Autodesk Inventor part; units mm, degrees
ref_plane "YZ Plane" through (0, 0, 0) normal (1, 0, 0) x (0, 1, 0)
ref_plane "XZ Plane" through (0, 0, 0) normal (0, 1, 0) x (-1, 0, 0)
ref_plane "XY Plane" through (0, 0, 0) normal (0, 0, 1) x (1, 0, 0)
sketch "Szkic1" plane through (0, 0, 0) normal (0, 0, 1) x (1, 0, 0)
  line L0 (-106, 20) -> (0, 20)
  line L1 (-106, 20) -> (-106, -2)
  line L2 (-106, -2) -> (24.7184, -2)
  line L3 (24.7184, -2) -> (24.7184, 3)
  line L4 (24.7184, 3) -> (0, 20)
  circle A0 centre (8, 6.2) radius 2 construction
  circle A1 centre (8, 6.2) radius 2.25
  line L5 (-57.5, 18) -> (-45.5, 18)
  line L6 (-45.5, 18) -> (-45.5, 8)
  line L7 (-45.5, 8) -> (-57.5, 8)
  line L8 (-57.5, 8) -> (-57.5, 18)
  line L9 (-70, 12.4) -> (-70, 0) construction
  arc A2 (-86.6773, 8.9692) -> (-86.6773, 3.4308) centre (-92, 6.2) ccw construction
  arc A3 (-86, 3.7) -> (-86, 8.7) centre (-86, 6.2) ccw construction
  arc A4 (-86.2337, 3.7) -> (-86.6773, 3.4308) centre (-86.2337, 3.2) ccw construction
  line L10 (-86.2337, 3.7) -> (-86, 3.7) construction
  arc A5 (-86.6773, 8.9692) -> (-86.2337, 8.7) centre (-86.2337, 9.2) ccw construction
  line L11 (-86, 8.7) -> (-86.2337, 8.7) construction
  arc A6 (-86.375, 8.9243) -> (-86.375, 3.4757) centre (-92, 6.2) ccw
  arc A7 (-86.375, 3.4757) -> (-86.375, 8.9243) centre (-86, 6.2) ccw
  line L12 (-116, 20) -> (-106, 20)
  line L13 (-106, 20) -> (-106, -2)
  line L14 (-106, -2) -> (-116, -2)
  line L15 (-116, -2) -> (-116, 20)
  line L16 (-92, 6.2) -> (-92, -8.9) construction
  line L17 (-92, -8.9) -> (-1, -8.9) construction
  line L18 (-72, -24) -> (-12, -24)
  line L19 (-12, -24) -> (-12, -2)
  line L20 (-12, -2) -> (-72, -2)
  line L21 (-72, -2) -> (-72, -24)
  point P0 (0, 0)
  point P1 (-7.9, -2)
  point P2 (-12, -2)
  dimension "d0" = 0.25
  dimension "d1" = 12.5
  dimension "d2" = 12
  dimension "d3" = 2
  dimension "d4" = 10
  dimension "d5" = 0.25
  dimension "d6" = 10
  dimension "d11" = 91
  dimension "d14" = 20
  dimension "d15" = 20
extrude "Wyciągnięcie proste1" add sketch "Szkic1" along normal blind 3
sketch "Szkic2" plane through (0, 0, 0) normal (0, 0, -1) x (-1, 0, 0)
  line L0 (12, -2) -> (18, -2)
  line L1 (18, -2) -> (18, -24)
  line L2 (18, -24) -> (12, -24)
  line L3 (12, -24) -> (12, -2)
  line L4 (66, -2) -> (72, -2)
  line L5 (72, -2) -> (72, -24)
  line L6 (72, -24) -> (66, -24)
  line L7 (66, -24) -> (66, -2)
  line L8 (72, -2) -> (72, -24)
  line L9 (12, -24) -> (12, -2)
  line L10 (72, -24) -> (12, -24)
  point P0 (0, 0)
  dimension "d16" = 6
  dimension "d17" = 6
extrude "Wyciągnięcie proste2" add sketch "Szkic2" along normal blind 20
sketch "Szkic4" plane through (-66, -24, 0) normal (1, 0, 0) x (0, 0, -1)
  line L0 (3, 18.7) -> (17, 18.7) construction
  line L1 (17, 18.7) -> (17, 3.3) construction
  line L2 (17, 3.3) -> (3, 3.3) construction
  line L3 (3, 3.3) -> (3, 18.7) construction
  line L4 (3, 18.7) -> (10, 11) construction
  line L5 (10, 11) -> (3, 3.3) construction
  line L6 (17, 3.3) -> (10, 11) construction
  line L7 (0, 22) -> (20, 22) construction
  line L8 (3, 18.7) -> (0, 22) construction
  line L9 (0, 0) -> (20, 0) construction
  line L10 (17, 3.3) -> (20, 0) construction
  line L11 (3, 3.3) -> (0, 0) construction
  line L12 (20, 22) -> (20, 0) construction
  point P0 (0, 24)
  dimension "d20" = 3
hole "Otwór2" at (-66, -13, -10) direction (-1, 0, 0) diameter 4.25 end through all both
sketch "Szkic5" plane through (-18, -24, 0) normal (-1, 0, 0) x (0, 0, 1)
  line L0 (-13.5, 11) -> (-13.5, 8.9793)
  line L1 (-13.5, 13.0207) -> (-13.5, 11)
  line L2 (-13.5, 8.9793) -> (-11.75, 7.9689)
  line L3 (-11.75, 7.9689) -> (-10, 6.9585)
  line L4 (-10, 6.9585) -> (-8.25, 7.9689)
  line L5 (-8.25, 7.9689) -> (-6.5, 8.9793)
  line L6 (-6.5, 8.9793) -> (-6.5, 11)
  line L7 (-6.5, 11) -> (-6.5, 13.0207)
  line L8 (-6.5, 13.0207) -> (-8.25, 14.0311)
  line L9 (-8.25, 14.0311) -> (-10, 15.0415)
  line L10 (-10, 15.0415) -> (-11.75, 14.0311)
  line L11 (-11.75, 14.0311) -> (-13.5, 13.0207)
  line L12 (-14, 8.6906) -> (-14, 11)
  line L13 (-14, 11) -> (-14, 13.3094)
  line L14 (-14, 13.3094) -> (-12, 14.4641)
  line L15 (-12, 14.4641) -> (-10, 15.6188)
  line L16 (-10, 15.6188) -> (-8, 14.4641)
  line L17 (-8, 14.4641) -> (-6, 13.3094)
  line L18 (-6, 13.3094) -> (-6, 11)
  line L19 (-6, 11) -> (-6, 8.6906)
  line L20 (-6, 8.6906) -> (-8, 7.5359)
  line L21 (-8, 7.5359) -> (-10, 6.3812)
  line L22 (-10, 6.3812) -> (-12, 7.5359)
  line L23 (-12, 7.5359) -> (-14, 8.6906)
  point P0 (0, 24)
  dimension "d36" = 0.5
extrude "Wyciągnięcie proste3" cut sketch "Szkic5" against normal blind 3 contours L1 L11 L10 L9 L8 L7 L6 L5 L4 L3 L2 L0 | L12 L13 L14 L15 L16 L17 L18 L19 L20 L21 L22 L23
sketch "Szkic6" plane through (-66, -24, 0) normal (1, 0, 0) x (0, 0, -1)
  line L0 (14, 8.6906) -> (14, 13.3094)
  line L1 (14, 13.3094) -> (10, 15.6188)
  line L2 (10, 15.6188) -> (6, 13.3094)
  line L3 (6, 13.3094) -> (6, 8.6906)
  line L4 (6, 8.6906) -> (10, 6.3812)
  line L5 (10, 6.3812) -> (14, 8.6906)
  point P0 (0, 24)
extrude "Wyciągnięcie proste4" cut sketch "Szkic6" against normal blind 3
sketch "Szkic7" plane through (0, 0, 3) normal (0, 0, 1) x (1, 0, 0)
  line L0 (-116, 20) -> (-116, -2)
  line L1 (-116, 20) -> (-106, 20)
  line L2 (-106, -2) -> (-116, -2)
  line L3 (-106, 20) -> (-106, -2)
  line L4 (0, 20) -> (-116, 20) construction
  line L5 (-116, 20) -> (-111, 9) construction
  line L6 (-111, 9) -> (-106, -2) construction
  line L7 (-116, -2) -> (-72, -2) construction
  line L8 (-116, -2) -> (-111, 9) construction
  point P0 (0, 0)
hole "Otwór3" at (-111, 9, 3) direction (0, 0, -1) diameter 4.25 end through all
sketch "Szkic8" plane through (0, 0, 0) normal (0, 0, -1) x (-1, 0, 0)
  line L0 (66, -18) -> (18, -18)
  line L1 (18, -18) -> (18, -24)
  line L2 (18, -24) -> (66, -24)
  line L3 (66, -24) -> (66, -18)
  line L4 (66, -2) -> (18, -2)
  line L5 (18, -2) -> (18, -8)
  line L6 (18, -8) -> (66, -8)
  line L7 (66, -8) -> (66, -2)
  line L8 (66, -24) -> (18, -24)
  point P0 (0, 0)
  dimension "d48" = 6
  dimension "d49" = 6
extrude "Wyciągnięcie proste5" add sketch "Szkic8" along normal blind 20
hole "Otwór1" at (-66, -5.3, -3) at (-66, -20.7, -17) at (-66, -20.7, -3) at (-66, -5.3, -17) direction (-1, 0, 0) diameter 2.75 end through all both
equation "\"d15\" = d14"
equation "\"d17\" = d16"
equation "\"d49\" = d48"
properties part number "wheel-adapter"
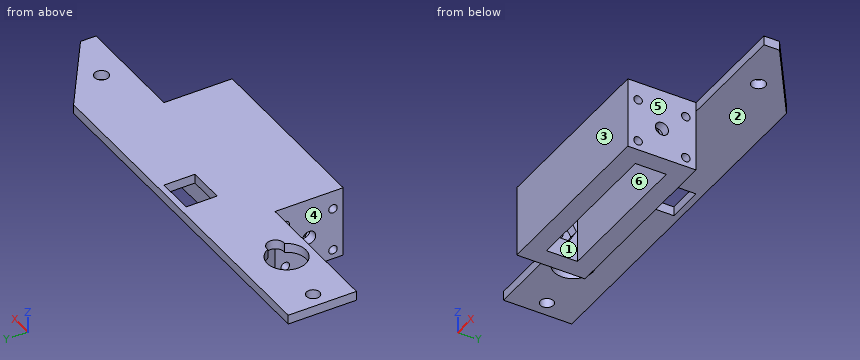
Verification items for the finished model (mm, model axes). Face numbers are marked on the shaded views. A direction names the side the tool comes from. Give positions to 0.01 mm unless a question says otherwise; leave off trailing zeros. Order: outer loops, then holes, each group sorted by start corner. A loop starts at its lowest first (then second) coordinate and runs counter-clockwise, first axis right, second up. Notation, with made-up numbers: M -22.5,84.5 L -17.5,84.5 A38 ccw -17.5,123.5 Z; hole C 29,24 d6. An arc over 180 degrees is marked long. Answer in a Markdown table with one row per item. Add a question column.
Item 1: Section check C-C, the plane y = -13. Enter the section's corners in (x, z) (3 decimals), and give its area (4 significant figures).
Item 2: Tool access check on the marked faces 4, 5 and 6. Record the directions out of +Z, -Z, +X, -X, +Y, -Y that give a thin tool (end or side, any length) a straight path to the whole face; none if there is none.
Item 3: Gauge pin test, flat ends, axial feed: pin 1 (3.5 mm diameter, centred on y = -5.3, z = -17, fed in from +X); pin 2 (20 mm diameter, centred on x = -92, y = 6.2, fed in from +Z); pin 3 (1.5 mm diameter, centred on x = 3, z = 2, fed in from -Y); pin 4 (3.5 mm diameter, centred on y = 11, z = 1, fed in from +X). Record the tip position at first contact, or that the pin passes through.
Item 4: Section check D-D, the plane x = -40.5. Enter the section's corners in (y, z) (3 decimals).
Item 5: Scan lines: probe 1 along Y at (x, z) = (-50.5, -3) (3 decimals); probe 2 along Z at (x, y) = (-57.5, -20.7) (3 decimals); probe 3 along Y at (x, z) = (-111, 1.05) (3 decimals). Record each from-to range of solid material in increasing order. Write a range as from..to.
Item 6: Section check B-B, the plane x = -92. Enter the section's corners in (y, z).
Item 7: Mould release check, pull along Y, two halves, no side actions. Record for the marked faces 1, 2 and 3: released by +Y, released by -Y, zero draft, split by the parting line, or undercut.
Item 8: Section check A-A, the plane z = -17. Enter the section's corners in (x, y) (3 decimals), and give its area (3 significant figures).
Filled sheet:
| question | item | result |
|---|---|---|
| 1 | outline | M -72,-20 L -66,-20 L -66,-14 L -69,-14 L -69,-12.125 L -72,-12.125 Z; M -72,-7.875 L -69,-7.875 L -69,-6 L -66,-6 L -66,0 L -18,0 L -18,-6 L -15,-6 L -15,-7.875 L -12,-7.875 L -12,3 L -72,3 Z; M -18,-20 L -12,-20 L -12,-12.125 L -15,-12.125 L -15,-14 L -18,-14 Z |
| 1 | area | 346.5 mm^2 |
| 2 | face 4 | +Z, -Z, -X, -Y |
| 2 | face 5 | +Z, -Z, +X, -Y |
| 2 | face 6 | -Z |
| 3 | pin 1 | stops at x = -12 |
| 3 | pin 2 | stops at z = 3 |
| 3 | pin 3 | stops at y = -2 |
| 3 | pin 4 | stops at x = 15.63 |
| 4 | outline | M -24,-20 L -18,-20 L -18,0 L -8,0 L -8,-20 L -2,-20 L -2,0 L 20,0 L 20,3 L -24,3 Z; hole C -20.7,-17 d2.75; hole C -20.7,-3 d2.75; hole C -5.3,-17 d2.75; hole C -5.3,-3 d2.75 |
| 5 | probe 1 | y = -24..-22.075, -19.325..-18, -8..-6.675, -3.925..-2 |
| 5 | probe 2 | z = -20..-18.375, -15.625..-4.375, -1.625..3 |
| 5 | probe 3 | y = -2..6.875, 11.125..20 |
| 6 | outline | M -2,0 L -0.05,0 L -0.05,3 L -2,3 Z; M 12.45,0 L 20,0 L 20,3 L 12.45,3 Z |
| 7 | face 1 | undercut |
| 7 | face 2 | zero draft |
| 7 | face 3 | released by -Y |
| 8 | outline | M -72,-24 L -12,-24 L -12,-22.075 L -72,-22.075 Z; M -72,-19.325 L -12,-19.325 L -12,-6.675 L -72,-6.675 Z; M -72,-3.925 L -12,-3.925 L -12,-2 L -72,-2 Z; hole M -66,-18 L -18,-18 L -18,-8 L -66,-8 Z |
| 8 | area | 510 mm^2 |
